```python
from build123d import *

# Parameters (mm, degrees)
BOSS_EXTRUDE3_DEPTH = 8
SKETCH3_R           = 2.1
CUT_EXTRUDE2_DEPTH  = 10
CUT_EXTRUDE3_REACH  = 10
SKETCH5_R           = 3
SKETCH5_R_2         = 7.5
SKETCH5_R_3         = 2.6
CUT_EXTRUDE4_REACH  = 10
SKETCH6_R           = 1.25


with BuildPart() as part:
    # Sketch1 → Boss-Extrude3 (new body)
    with BuildSketch(Plane(origin=(0, 0, 0), x_dir=(1, 0, 0), z_dir=(0, 1, 0))):
        Polygon((40.5, -35), (56.816666667, -90), (82, -90), (82, 90), (-82, 90), (-82, -90), (-56.816666667, -90), (-40.5, -35), align=None)
    extrude(amount=BOSS_EXTRUDE3_DEPTH)

    # Sketch3 → Cut-Extrude2 (cut)
    with BuildSketch(Plane(origin=(-73, 8, 0), x_dir=(0, 0, 1), z_dir=(0, 1, 0))):
        with Locations((-45.25, -5)):
            Circle(SKETCH3_R)
        with Locations((-86, -5)):
            Circle(SKETCH3_R)
        with Locations((-86, 34)):
            Circle(SKETCH3_R)
        with Locations((-86, 73)):
            Circle(SKETCH3_R)
        with Locations((-86, 112)):
            Circle(SKETCH3_R)
        with Locations((-86, 151)):
            Circle(SKETCH3_R)
        with Locations((-4.5, -5)):
            Circle(SKETCH3_R)
        with Locations((-4.5, 151)):
            Circle(SKETCH3_R)
        with Locations((-45.25, 151)):
            Circle(SKETCH3_R)
        with Locations((86, 7.59)):
            Circle(SKETCH3_R)
        with Locations((86, 138.41)):
            Circle(SKETCH3_R)
    extrude(amount=-CUT_EXTRUDE2_DEPTH, mode=Mode.SUBTRACT)

    # Sketch5 → Cut-Extrude3 (cut, up to next)
    with BuildSketch(Plane(origin=(0, 8, 0), x_dir=(1, 0, 0), z_dir=(0, 1, 0)), mode=Mode.PRIVATE) as cut_extrude3_sk1:
        with Locations((62, -74.75)):
            Circle(SKETCH5_R)
    cut_extrude3_tool1 = extrude(cut_extrude3_sk1.sketch, amount=-CUT_EXTRUDE3_REACH, mode=Mode.PRIVATE) & part.part
    add(cut_extrude3_tool1.solids().sort_by_distance((62, 8, 74.75))[0], mode=Mode.SUBTRACT)
    # Sketch5 → Cut-Extrude3 (cut, up to next)
    with BuildSketch(Plane(origin=(0, 8, 0), x_dir=(1, 0, 0), z_dir=(0, 1, 0)), mode=Mode.PRIVATE) as cut_extrude3_sk2:
        with Locations((62, -19.99)):
            Circle(SKETCH5_R)
    cut_extrude3_tool2 = extrude(cut_extrude3_sk2.sketch, amount=-CUT_EXTRUDE3_REACH, mode=Mode.PRIVATE) & part.part
    add(cut_extrude3_tool2.solids().sort_by_distance((62, 8, 19.99))[0], mode=Mode.SUBTRACT)
    # Sketch5 → Cut-Extrude3 (cut, up to next)
    with BuildSketch(Plane(origin=(0, 8, 0), x_dir=(1, 0, 0), z_dir=(0, 1, 0)), mode=Mode.PRIVATE) as cut_extrude3_sk3:
        with Locations((-62, -74.75)):
            Circle(SKETCH5_R)
    cut_extrude3_tool3 = extrude(cut_extrude3_sk3.sketch, amount=-CUT_EXTRUDE3_REACH, mode=Mode.PRIVATE) & part.part
    add(cut_extrude3_tool3.solids().sort_by_distance((-62, 8, 74.75))[0], mode=Mode.SUBTRACT)
    # Sketch5 → Cut-Extrude3 (cut, up to next)
    with BuildSketch(Plane(origin=(0, 8, 0), x_dir=(1, 0, 0), z_dir=(0, 1, 0)), mode=Mode.PRIVATE) as cut_extrude3_sk4:
        with Locations((-62, -19.99)):
            Circle(SKETCH5_R)
    cut_extrude3_tool4 = extrude(cut_extrude3_sk4.sketch, amount=-CUT_EXTRUDE3_REACH, mode=Mode.PRIVATE) & part.part
    add(cut_extrude3_tool4.solids().sort_by_distance((-62, 8, 19.99))[0], mode=Mode.SUBTRACT)
    # Sketch5 → Cut-Extrude3 (cut, up to next)
    with BuildSketch(Plane(origin=(0, 8, 0), x_dir=(1, 0, 0), z_dir=(0, 1, 0)), mode=Mode.PRIVATE) as cut_extrude3_sk5:
        with Locations((0, -6.25)):
            Circle(SKETCH5_R_2)
    cut_extrude3_tool5 = extrude(cut_extrude3_sk5.sketch, amount=-CUT_EXTRUDE3_REACH, mode=Mode.PRIVATE) & part.part
    add(cut_extrude3_tool5.solids().sort_by_distance((0, 8, 6.25))[0], mode=Mode.SUBTRACT)
    # Sketch5 → Cut-Extrude3 (cut, up to next)
    with BuildSketch(Plane(origin=(0, 8, 0), x_dir=(1, 0, 0), z_dir=(0, 1, 0)), mode=Mode.PRIVATE) as cut_extrude3_sk6:
        with Locations((0, -22.5)):
            Circle(SKETCH5_R_3)
    cut_extrude3_tool6 = extrude(cut_extrude3_sk6.sketch, amount=-CUT_EXTRUDE3_REACH, mode=Mode.PRIVATE) & part.part
    add(cut_extrude3_tool6.solids().sort_by_distance((0, 8, 22.5))[0], mode=Mode.SUBTRACT)

    # Sketch6 → Cut-Extrude4 (cut, up to next)
    with BuildSketch(Plane(origin=(0, 8, 0), x_dir=(1, 0, 0), z_dir=(0, 1, 0)), mode=Mode.PRIVATE) as cut_extrude4_sk1:
        with Locations((-56, 8.5)):
            Circle(SKETCH6_R)
    cut_extrude4_tool1 = extrude(cut_extrude4_sk1.sketch, amount=-CUT_EXTRUDE4_REACH, mode=Mode.PRIVATE) & part.part
    add(cut_extrude4_tool1.solids().sort_by_distance((-56, 8, -8.5))[0], mode=Mode.SUBTRACT)
    # Sketch6 → Cut-Extrude4 (cut, up to next)
    with BuildSketch(Plane(origin=(0, 8, 0), x_dir=(1, 0, 0), z_dir=(0, 1, 0)), mode=Mode.PRIVATE) as cut_extrude4_sk2:
        with Locations((-56, 50)):
            Circle(SKETCH6_R)
    cut_extrude4_tool2 = extrude(cut_extrude4_sk2.sketch, amount=-CUT_EXTRUDE4_REACH, mode=Mode.PRIVATE) & part.part
    add(cut_extrude4_tool2.solids().sort_by_distance((-56, 8, -50))[0], mode=Mode.SUBTRACT)
    # Sketch6 → Cut-Extrude4 (cut, up to next)
    with BuildSketch(Plane(origin=(0, 8, 0), x_dir=(1, 0, 0), z_dir=(0, 1, 0)), mode=Mode.PRIVATE) as cut_extrude4_sk3:
        with Locations((56, 50)):
            Circle(SKETCH6_R)
    cut_extrude4_tool3 = extrude(cut_extrude4_sk3.sketch, amount=-CUT_EXTRUDE4_REACH, mode=Mode.PRIVATE) & part.part
    add(cut_extrude4_tool3.solids().sort_by_distance((56, 8, -50))[0], mode=Mode.SUBTRACT)
    # Sketch6 → Cut-Extrude4 (cut, up to next)
    with BuildSketch(Plane(origin=(0, 8, 0), x_dir=(1, 0, 0), z_dir=(0, 1, 0)), mode=Mode.PRIVATE) as cut_extrude4_sk4:
        with Locations((56, 8.5)):
            Circle(SKETCH6_R)
    cut_extrude4_tool4 = extrude(cut_extrude4_sk4.sketch, amount=-CUT_EXTRUDE4_REACH, mode=Mode.PRIVATE) & part.part
    add(cut_extrude4_tool4.solids().sort_by_distance((56, 8, -8.5))[0], mode=Mode.SUBTRACT)


solid = part.part
```
Source: CAD feature listing. Evaluate the final solid. Frame: model axes, mm. A direction names the side the tool comes from. Round coordinates to 2 decimals unless told otherwise and drop trailing zeros. Loops run counter-clockwise (first coordinate to the right, second up) from the corner with the lowest first, then second, coordinate; pieces in that order, holes last.
1. Contact query for a flat-ended pin moving along its axis: pin 1 (9.5 mm diameter, centred on x = -62, z = 19.99, fed in from -Y). Output: stop coordinate, or through.
2. Access query for faces 1 (the flat face through (-1, 4, 35)), 2 (the cylindrical face through (-64.381, 4.056, 76.575)). Directions: +Z, -Z, +X, -X, +Y, -Y. A direction counts if a zero-diameter tool reaches every point of the face in a straight line with its end or side. Return the directions, or none.
3. Section query A-A on x = 0. Output: boundary loops of the cut face in (y, z).
4. Section query D-D on x = -43.5. Output: boundary loops of the cut face in (y, z), and give its area (3 significant figures).
5. Section query C-C on z = 64. Output: boundary loops of the cut face in (x, y).
6. Ray query, L1, parallel to X at y = 2.5, z = -45.25; L2, parallel to Z at x = 62, y = 2.75; L3, parallel to X at y = 5, z = 19. Return the intervals inside material, ascending.
7. Section query B-B on y = 1.25. Give the number of separate pieces and of enclosed holes in the cut face, and give its area (3 significant figures).
8. Mould query, pull axis X, two halves, no side actions, for faces 3 (the flat face through (-1, 0, -21)), 4 (the cylindrical face through (78.09, 4.06, -88.1)). Classes: released by +X, released by -X, zero draft, split by the parting line, or undercut.
Answers below:
1. pin 1: stops at y = 0
2. face 1: +Z, +Y, -Y
2. face 2: +Y, -Y
3. outline: (0, -90) - (8, -90) - (8, -88.1) - (0, -88.1) - close; (0, -83.9) - (8, -83.9) - (8, -1.25) - (0, -1.25) - close; (0, 13.75) - (8, 13.75) - (8, 19.9) - (0, 19.9) - close; (0, 25.1) - (8, 25.1) - (8, 35) - (0, 35) - close
4. outline: (0, -90) - (8, -90) - (8, 45.11) - (0, 45.11) - close
4. area: 1,080 mm2
5. outline: (-82, 0) - (-49.1, 0) - (-49.1, 8) - (-82, 8) - close; (49.1, 0) - (82, 0) - (82, 8) - (49.1, 8) - close
6. L1: x = -82 to -80.1, -75.9 to 75.9, 80.1 to 82
6. L2: z = -90 to 16.99, 22.99 to 71.75, 77.75 to 90
6. L3: x = -82 to -64.83, -59.17 to 59.17, 64.83 to 82
7. separate pieces: 1
7. enclosed holes: 21
7. area: 23,700 mm2
8. face 3: zero draft
8. face 4: undercut
